Could you check a few things on this model? Use its own coordinates, in mm. A direction names the side the tool comes from. Give positions to 0.01 mm unless a question says otherwise; leave off trailing zeros. Loops run counter-clockwise (first coordinate to the right, second up) from the corner with the lowest first, then second, coordinate; pieces in that order, holes last. Notation, with made-up numbers: (-30, 72) -> (11, 72) arc R34 ccw to (11, 108) -> close; hole circle Ø11 at (4.25, 25). An arc over 180 degrees is marked (long way). Write each question's results on one line, items separated by ' | '. Start each with the question number.
Q1. Which directions (+Z, -Z, +X, -X, +Y, -Y) give clear straight access to the entire face, cutting with the end or side of a thin tool? Please do faces 4 (the face through (-4.5, -1.8, 0.1)), 5 (the face through (0, -3.5, 0)).
Q2. If I drill on line 1 along X through (y, z) = (-0.85, 0.25); line 2 along X through (y, z) = (-1.55, -2); line 3 along Z through (x, y) = (-3.25, -1.85), over which ranges is the centre line in solid material (lowest first)?
Q3. If we section it at A-A, the plane z = 0: List the corners of the cut face in (x, y) for me, plus the area to 3 significant figures.
Q4. Will these pins go through, and if not, where does the flat tip stop? P1, Ø1, axis at x = 4.5, y = -1.5, coming from the -Z side; P2, Ø1.5, axis at y = -1, z = 2, coming from the +X side; P3, Ø2, axis at x = -1.5, y = -1, coming from the -Z side.
Q5. We'd pull the mould along X, two halves only. Please class faces 1 (the face through (4.5, -1.8, -0.1)), 2 (the face through (-7.493, -1.726, 0.33)), 3 (the face through (0, 0, 0)): released by +X, released by -X, zero draft, split by the parting line, or undercut.
Q6. If we section it at D-D, the plane x = -1.75: List the corners of the cut face in (y, z) for me, plus the area to 3 significant figures.
Q7. If we section it at C-C, the plane y = -2.35: List the corners of the cut face in (x, z) for me.
Q8. If we section it at B-B, the plane x = -3.75: List the corners of the cut face in (y, z) for me, plus the area to 3 significant figures.
from build123d import *

# Parameters (mm, degrees)
F0_R     = 7.5
F1_DEPTH = 3.5
F3_DEPTH = 25


with BuildPart() as f1:
    # F0 (on Front) → F1 (new body)
    with BuildSketch(Plane.XZ):
        Circle(F0_R)
    extrude(amount=F1_DEPTH)

    # F2 (on face) → F3 (cut)
    with BuildSketch(Plane.XZ.offset(3.5)):
        with BuildLine():
            ThreePointArc((1.5, -3), (4.5, 0), (1.5, 3))
            Line((1.5, 3), (1.5, -3))
        make_face()
        with BuildLine():
            Line((-1.5, -3), (-1.5, 3))
            ThreePointArc((-1.5, 3), (-4.5, 0), (-1.5, -3))
        make_face()
    extrude(amount=-F3_DEPTH, mode=Mode.SUBTRACT)


solid = f1.part
Final values:
1) face 4: +Y, -Y | face 5: +Z, -Z, +X, -X, -Y
2) line 1: x = -7.5 to -4.49, -1.5 to 1.5, 4.49 to 7.5 | line 2: x = -7.23 to -3.74, -1.5 to 1.5, 3.74 to 7.23 | line 3: z = -6.76 to -2.44, 2.44 to 6.76
3) outline: (-7.5, -3.5) -> (-4.5, -3.5) -> (-4.5, 0) -> (-7.5, 0) -> close; (-1.5, -3.5) -> (1.5, -3.5) -> (1.5, 0) -> (-1.5, 0) -> close; (4.5, -3.5) -> (7.5, -3.5) -> (7.5, 0) -> (4.5, 0) -> close | area: 31.5 mm²
4) P1: stops at z = -6.34 | P2: stops at x = 7.4 | P3: stops at z = -7.48
5) face 1: undercut | face 2: split by the parting line | face 3: zero draft
6) outline: (-3.5, -7.29) -> (0, -7.29) -> (0, -2.99) -> (-3.5, -2.99) -> close; (-3.5, 2.99) -> (0, 2.99) -> (0, 7.29) -> (-3.5, 7.29) -> close | area: 30.1 mm²
7) outline: circle Ø15 at (0, 0); hole (-1.5, -3) -> (-1.5, 3) arc R3 ccw to start; hole (1.5, -3) arc R3 ccw to (1.5, 3) -> close
8) outline: (-3.5, -6.5) -> (0, -6.5) -> (0, -1.98) -> (-3.5, -1.98) -> close; (-3.5, 1.98) -> (0, 1.98) -> (0, 6.5) -> (-3.5, 6.5) -> close | area: 31.6 mm²
